Part model, mm, in its own coordinate system. A direction names the side the tool comes from. Coordinates: 2 decimals unless noted, no trailing zeros. Loops run counter-clockwise (first coordinate to the right, second up) from the corner with the lowest first, then second, coordinate; pieces in that order, holes last.
```python
from build123d import *

# Parameters (mm, degrees)
F0_W      = 100
F0_H      = 100
F1_DEPTH  = 96
F2_W      = 17.5
F2_H      = 78
F3_DEPTH  = 100.001
F4_W      = 65
F4_H      = 78
F5_DEPTH  = 45
F6_W      = 65
F6_H      = 78
F7_DEPTH  = 10
F8_W      = 65
F8_H      = 73
F9_DEPTH  = 15
F11_DEPTH = 100.001
F12_R     = 1.5
F12_R_2   = 2
F13_DEPTH = 10
F14_R     = 2
F15_DEPTH = 8


with BuildPart() as f1:
    # F0 (on Front) → F1 (new body)
    with BuildSketch(Plane.XZ):
        with Locations((0, 50)):
            Rectangle(F0_W, F0_H)
    extrude(amount=-F1_DEPTH)

    # F2 (on face) → F3 (cut, through all)
    with BuildSketch(Plane.XY.offset(100)):
        with Locations((-41.25, 57)):
            Rectangle(F2_W, F2_H)
        with Locations((41.25, 57)):
            Rectangle(F2_W, F2_H)
        Polygon((-22.5, 74), (-22.5, 18), (22.5, 18), (22.5, 74), (16, 74), (16, 86), (-16, 86), (-16, 74), align=None)
    extrude(amount=-F3_DEPTH, mode=Mode.SUBTRACT)

    # F4 (on face) → F5 (cut)
    with BuildSketch(Plane.XY.offset(100)):
        with Locations((0, 57)):
            Rectangle(F4_W, F4_H)
    extrude(amount=-F5_DEPTH, mode=Mode.SUBTRACT)

    # F6 (on face) → F7 (cut)
    with BuildSketch(Plane(origin=(0, 0, 0), x_dir=(1, 0, 0), z_dir=(0, 0, -1))):
        with Locations((0, -57)):
            Rectangle(F6_W, F6_H)
    extrude(amount=-F7_DEPTH, mode=Mode.SUBTRACT)

    # F8 (on face) → F9 (cut)
    with BuildSketch(Plane.XY.offset(55)):
        with Locations((0, 59.5)):
            Rectangle(F8_W, F8_H)
    extrude(amount=-F9_DEPTH, mode=Mode.SUBTRACT)

    # F10 (on face) → F11 (cut, through all)
    with BuildSketch(Plane.YZ.offset(50)):
        Polygon((0, 18), (0, 10), (5, 10), (5, 7), (10, 7), (10, 21), (5, 21), (5, 18), align=None)
        Polygon((5, 46), (5, 43), (10, 43), (10, 57), (5, 57), (5, 54), (0, 54), (0, 46), align=None)
        Polygon((5, 82), (5, 79), (10, 79), (10, 93), (5, 93), (5, 90), (0, 90), (0, 82), align=None)
    extrude(amount=-F11_DEPTH, mode=Mode.SUBTRACT)

    # F12 (on face) → F13 (cut)
    with BuildSketch(Plane(origin=(0, 96, 0), x_dir=(-1, 0, 0), z_dir=(0, 1, 0))):
        with Locations((-12.5, 35)):
            Circle(F12_R)
        with Locations((-12.5, 15)):
            Circle(F12_R)
        with Locations((12.5, 35)):
            Circle(F12_R)
        with Locations((12.5, 15)):
            Circle(F12_R)
        with Locations((0, 25)):
            Circle(F12_R_2)
    extrude(amount=-F13_DEPTH, mode=Mode.SUBTRACT)

    # F14 (on face) → F15 (cut)
    with BuildSketch(Plane(origin=(0, 18, 0), x_dir=(-1, 0, 0), z_dir=(0, 1, 0))):
        with Locations((18, 50.5)):
            Circle(F14_R)
        with Locations((18, 14.5)):
            Circle(F14_R)
        with Locations((-18, 50.5)):
            Circle(F14_R)
        with Locations((-18, 14.5)):
            Circle(F14_R)
    extrude(amount=-F15_DEPTH, mode=Mode.SUBTRACT)


solid = f1.part
```
Q1. Saw through at D-D (z = 50.5). List the corners of the cut face in (x, y).
Q2. Saw through at A-A (y = 28). List the corners of the cut face in (x, z), plus the area to 3 significant figures.
Q3. Mould opens along Z. For faces 1 (the flat face through (-1, 0, 5)), 2 (the flat face through (1, 5, 45)), 3 (the flat face through (27, 21, 55)), 4 (the flat face through (1, 5, 9)) say: released by +Z, released by -Z, zero draft, split by the parting line, or undercut.
Q4. Probe line 1 (Z direction, x = 18, y = 16); line 2 (Z direction, x = -39, y = 6); line 3 (Z direction, x = 12.5, y = 93). List the from-to ranges inside material, lowest first.
Q5. Tool access for faces 5 (the flat face through (1, 3, 90)), 6 (the flat face through (0, 86, 29)), 7 (the cylindrical face through (18.26, 14.056, 16.483)), 8 (the flat face through (-28, 23, 48)), 9 (the flat face through (1, 10, 86)): list every direction of +Z, -Z, +X, -X, +Y, -Y with a clear straight run to the whole face (end or side of a thin tool).
Q6. Drop flat-ended pins along their axis: P1, Ø8, axis at x = -30, z = 52, coming from the -Y side; P2, Ø12, axis at x = -16.5, z = 72, coming from the +Y side; P3, Ø4, axis at x = 27.5, y = 20.5, coming from the +Z side; P4, Ø8, axis at x = -27, z = 47.5, coming from the +Y side. Give the stop position or say it passes through.
Q7. Saw through at C-C (z = 35). List the corners of the cut face in (x, y), plus the area to 3 significant figures.
Q8. Saw through at B-B (y = 88.5). List the corners of the cut face in (x, z), plus the area to 3 significant figures.
Checked values:
1. outline: (-50, 10) - (-20, 10) - (-20, 18) - (-22.5, 18) - (-22.5, 23) - (-32.5, 23) - (-32.5, 18) - (-50, 18) - close; (-16, 10) - (16, 10) - (16, 18) - (-16, 18) - close; (20, 10) - (50, 10) - (50, 18) - (32.5, 18) - (32.5, 23) - (22.5, 23) - (22.5, 18) - (20, 18) - close
2. outline: (-32.5, 10) - (-22.5, 10) - (-22.5, 40) - (-32.5, 40) - close; (22.5, 10) - (32.5, 10) - (32.5, 40) - (22.5, 40) - close
2. area: 600 mm2
3. face 1: zero draft
3. face 2: undercut
3. face 3: released by +Z
3. face 4: undercut
4. line 1: z = 0 to 12.5, 16.5 to 48.5, 52.5 to 100
4. line 2: z = 0 to 7, 21 to 43, 57 to 79, 93 to 100
4. line 3: z = 10 to 13.5, 16.5 to 33.5, 36.5 to 40
5. face 5: +X, -X, -Y
5. face 6: +Z, -Z
5. face 7: -Y
5. face 8: +Z, +X, -X, +Y
5. face 9: +X, -X
6. P1: stops at y = 0
6. P2: stops at y = 18
6. P3: stops at z = 55
6. P4: stops at y = 23
7. outline: (-50, 0) - (50, 0) - (50, 18) - (32.5, 18) - (32.5, 96) - (14, 96) - (14, 86) - (16, 86) - (16, 74) - (22.5, 74) - (22.5, 18) - (-22.5, 18) - (-22.5, 74) - (-16, 74) - (-16, 86) - (-14, 86) - (-14, 96) - (-32.5, 96) - (-32.5, 18) - (-50, 18) - close; (-11, 86) - (11, 86) - (11, 96) - (-11, 96) - close
7. area: 3,910 mm2
8. outline: (-32.5, 10) - (32.5, 10) - (32.5, 40) - (-32.5, 40) - close; hole circle Ø3 at (-12.5, 15); hole circle Ø3 at (-12.5, 35); hole circle Ø4 at (0, 25); hole circle Ø3 at (12.5, 15); hole circle Ø3 at (12.5, 35)
8. area: 1,910 mm2
